```python
from build123d import *

# Parameters (mm, degrees)
F1_DEPTH  = 20
F2_R      = 2.5
F3_DEPTH  = 24.001
F4_SIZE   = 0.5
F5_R      = 2.5
F6_DEPTH  = 28.5
F8_DEPTH  = 4
F10_DEPTH = 4
F11_SIZE  = 1.5


with BuildPart() as f1:
    # F0 (on Top) → F1 (new body)
    with BuildSketch(Plane.XY):
        Polygon((0, 4), (0, 0), (70, 0), (70, 4), (49.25, 4), (49.25, 24), (45.25, 24), (45.25, 18.5), (44.75, 18), (44.75, 10), (45.25, 9.5), (45.25, 4), (39.75, 4), (38.25, 5.5), (32.25, 5.5), (30.75, 4), (24.75, 4), (24.75, 9.5), (25.25, 10), (25.25, 18), (24.75, 18.5), (24.75, 24), (20.75, 24), (20.75, 4), align=None)
    extrude(amount=F1_DEPTH)

    # F2 (on face) → F3 (cut, through all)
    with BuildSketch(Plane.XZ):
        with Locations((10, 10)):
            Circle(F2_R)
        with Locations((60, 10)):
            Circle(F2_R)
    extrude(amount=-F3_DEPTH, mode=Mode.SUBTRACT)

    # F4
    f4_edges = [f1.edges().sort_by_distance(p)[0] for p in [
        (25.25, 14, 20),
        (25.25, 14, 0),
        (44.75, 14, 20),
        (44.75, 14, 0),
    ]]
    chamfer(f4_edges, length=F4_SIZE)

    # F5 (on face) → F6 (cut, through all)
    with BuildSketch(Plane.YZ.offset(49.25)):
        with Locations((14, 10)):
            Circle(F5_R)
    extrude(amount=-F6_DEPTH, mode=Mode.SUBTRACT)

    # F7 (on face) → F8 (join)
    with BuildSketch(Plane.XY.offset(20)):
        Polygon((20.75, 4), (20.75, 24), (0, 4), align=None)
        Polygon((70, 4), (49.25, 24), (49.25, 4), align=None)
    extrude(amount=-F8_DEPTH)

    # F9 (on face) → F10 (join)
    with BuildSketch(Plane(origin=(0, 0, 0), x_dir=(1, 0, 0), z_dir=(0, 0, -1))):
        Polygon((0, -4), (20.75, -24), (20.75, -4), align=None)
        Polygon((49.25, -24), (70, -4), (49.25, -4), align=None)
    extrude(amount=-F10_DEPTH)

    # F11
    f11_edges = [f1.edges().sort_by_distance(p)[0] for p in [
        (35.25, 5.5, 20),
        (35.25, 5.5, 0),
    ]]
    chamfer(f11_edges, length=F11_SIZE)


solid = f1.part
```
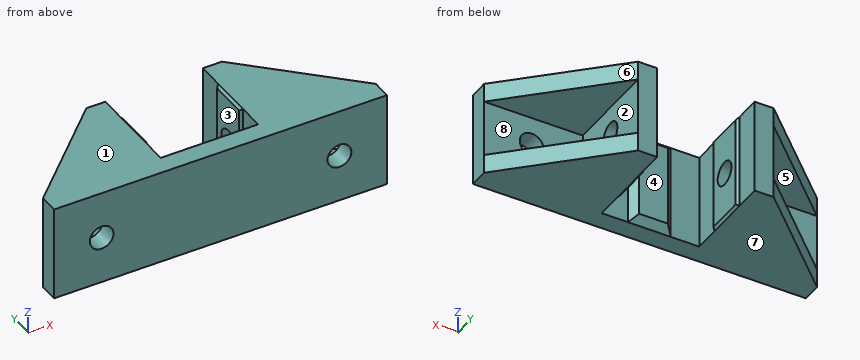
Here's how the part is built. I have some questions about the finished solid (model axes, mm). Face numbers are marked on the shaded views. A direction names the side the tool comes from. Coordinates: 2 decimals unless noted, no trailing zeros. Write each loop counter-clockwise with the first axis right and the second up, starting at its lowest first coordinate (ties: lowest second). Pieces come first, ordered by that corner, then holes. Notation, with made-up numbers: M -27,64.25 L -8,64.25 A28 cw -8,100.25 Z; hole C 43.25,-32.75 d2. An arc over 180 degrees is marked long. Answer as CSV lines item,"result". Start each with the question number.
Q1. For the marked faces 4, 5, 6, 7 and 8, which set-ups out of +Z, -Z, +X, -X, +Y, -Y let a thin tool reach every point of the face, with its end or its side?
Q2. Suppose I cut it at D-D, the plane x = 31.5. List the corners of the cut face in (y, z) for me, then the cut area to 3 significant figures.
Q3. If we mould it in two halves opening along Z, with no side actions, what happens to the marked faces 1, 2 and 3? For each: pulls with the +Z half, pulls with the -Z half, needs draft (parallel to the pull), parting line crosses it, or undercut.
Q4. Suppose I cut it at B-B, the plane y = 14. List the corners of the cut face in (x, z) for me (3 decimals), then the cut area to 4 significant figures.
Q5. I need wall thicknesses on probe 1 along Z at (x, y) = (7.5, 9); probe 2 along Z at (x, y) = (45.95, 14); probe 3 along X at (y, z) = (16.75, 6). Which ranges of each line are inside material? Lowest first, please. Write a range as [from, to].
Q6. Will these pins go through, and if not, where does the flat tip stop? pin 1 Ø5 at (x, z) = (29, 13.5) entering from +Y; pin 2 Ø3 at (y, z) = (19, 16.5) entering from -X; pin 3 Ø6 at (y, z) = (13.5, 7.5) entering from -X; pin 4 Ø6 at (x, y) = (64, 14.5) entering from -Z.
Q7. Suppose I cut it at C-C, the plane x = 22. List the corners of the cut face in (y, z) for me, then the cut area to 3 significant figures.
Q8. Suppose I cut it at A-A, the plane z = 16.75. List the corners of the cut face in (x, y) for me, then the cut area to 3 significant figures.
Entries:
1,face 4,"+Z, -Z, +Y"
1,face 5,"-X, +Y"
1,face 6,"+Z, -Z, +X, +Y"
1,face 7,"-Z, +X, -X, +Y, -Y"
1,face 8,"+X, +Y"
2,outline,"M 0,0 L 4,0 L 4.75,0.75 L 4.75,19.25 L 4,20 L 0,20 Z"
2,area,"94.4 mm²"
3,face 1,"pulls with the +Z half"
3,face 2,"undercut"
3,face 3,"needs draft"
4,outline,"M 10.375,0 L 24.75,0 L 25.25,0.5 L 25.25,7.5 L 20.75,7.5 L 20.75,4 L 10.375,4 Z; M 10.375,16 L 20.75,16 L 20.75,12.5 L 25.25,12.5 L 25.25,19.5 L 24.75,20 L 10.375,20 Z; M 44.75,0.5 L 45.25,0 L 59.625,0 L 59.625,4 L 49.25,4 L 49.25,7.5 L 44.75,7.5 Z; M 44.75,12.5 L 49.25,12.5 L 49.25,16 L 59.625,16 L 59.625,20 L 45.25,20 L 44.75,19.5 Z"
4,area,"300.5 mm²"
5,probe 1,"z = [0, 4], [16, 20]"
5,probe 2,"z = [0, 7.5], [12.5, 20]"
5,probe 3,"x = [20.75, 25.25], [44.75, 49.25]"
6,pin 1,"stops at y = 4.75"
6,pin 2,"stops at x = 14.01"
6,pin 3,"stops at x = 20.75"
6,pin 4,"passes through"
7,outline,"M 0,0 L 24,0 L 24,20 L 0,20 Z; hole C 14,10 d5"
7,area,"460 mm²"
8,outline,"M 0,0 L 70,0 L 70,4 L 49.25,24 L 45.25,24 L 45.25,18.5 L 44.75,18 L 44.75,10 L 45.25,9.5 L 45.25,4 L 39.75,4 L 38.25,5.5 L 32.25,5.5 L 30.75,4 L 24.75,4 L 24.75,9.5 L 25.25,10 L 25.25,18 L 24.75,18.5 L 24.75,24 L 20.75,24 L 0,4 Z"
8,area,"875 mm²"
